Drawing for the job (mm, zero at the part's lowest x, y, z). A direction names the side the tool comes from. Coordinates: 2 decimals unless noted, no trailing zeros. Write each loop counter-clockwise with the first axis right and the second up, starting at its lowest first coordinate (ties: lowest second). Pieces come first, ordered by that corner, then holes. Notation, with made-up numbers: M 84.25,2.5 L 136.25,2.5 A19 ccw 136.25,19.5 Z; hole C -29.75,46 d7. An arc over 180 degrees is marked long. Put each result on its own line as item: value. Start each with the question number.
Q1. Pull direction Y, two halves, no side cores. Call the marked faces 1, 2 and 3: pulls with the +Y half, pulls with the -Y half, needs draft (parallel to the pull), parting line crosses it, or undercut.
Q2. Cut at B-B (x = 12.7). Write the cut outline in (y, z).
Q3. Cut at C-C (y = 12.7). Write the cut outline in (x, z).
Q4. Cut at A-A (y = 63.5). Write the cut outline in (x, z).
Q5. Cut at D-D (z = 1.75). Write the cut outline in (x, y).
Q6. Which spindle directions (+Z, -Z, +X, -X, +Y, -Y) get a long thin tool onto all of the face, cutting with end or side? Do the marked faces 4 and 5. Say none if no direction does.
Q7. Drop flat-ended pins along their axis: pin 1 (2 mm diameter, centred on y = 21, z = 2.5, fed in from -X); pin 2 (3 mm diameter, centred on x = 16.5, z = 3, fed in from -Y). Give the stop position or say it passes through.
Q8. Drill centre lines: line 1 along Y through (x, z) = (38.1, 3.25); line 2 along Y through (x, z) = (37.5, 1.25); line 3 along X through (y, z) = (5.5, 4). Where is each one in solid material? Low to high.
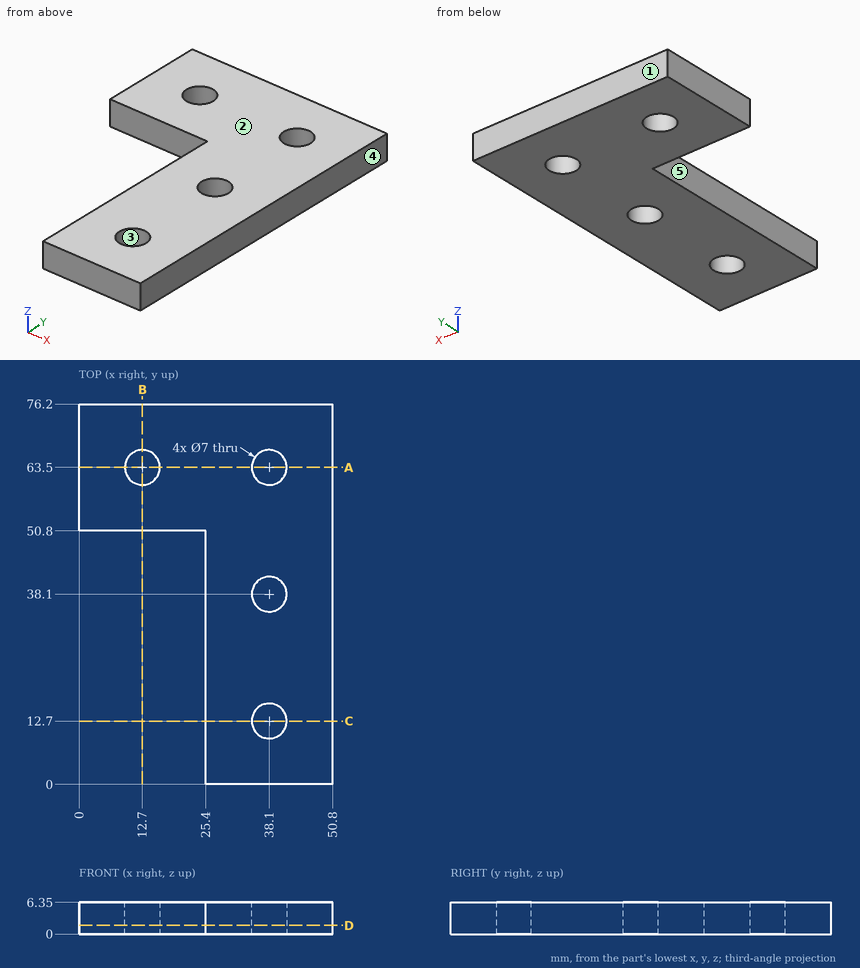
Computed values:
1. face 1: pulls with the +Y half
1. face 2: needs draft
1. face 3: undercut
2. outline: M 50.8,0 L 60,0 L 60,6.35 L 50.8,6.35 Z; M 67,0 L 76.2,0 L 76.2,6.35 L 67,6.35 Z
3. outline: M 25.4,0 L 34.6,0 L 34.6,6.35 L 25.4,6.35 Z; M 41.6,0 L 50.8,0 L 50.8,6.35 L 41.6,6.35 Z
4. outline: M 0,0 L 9.2,0 L 9.2,6.35 L 0,6.35 Z; M 16.2,0 L 34.6,0 L 34.6,6.35 L 16.2,6.35 Z; M 41.6,0 L 50.8,0 L 50.8,6.35 L 41.6,6.35 Z
5. outline: M 0,50.8 L 25.4,50.8 L 25.4,0 L 50.8,0 L 50.8,76.2 L 0,76.2 Z; hole C 12.7,63.5 d7; hole C 38.1,12.7 d7; hole C 38.1,38.1 d7; hole C 38.1,63.5 d7
6. face 4: +Z, -Z, +X, +Y, -Y
6. face 5: +Z, -Z, -X, -Y
7. pin 1: x = 25.4
7. pin 2: y = 50.8
8. line 1: 0 to 9.2, 16.2 to 34.6, 41.6 to 60, 67 to 76.2
8. line 2: 0 to 9.25, 16.15 to 34.65, 41.55 to 60.05, 66.95 to 76.2
8. line 3: 25.4 to 50.8
